Source: CAD feature listing. Evaluate the final solid. Frame: model axes, mm. A direction names the side the tool comes from. Coordinates: 2 decimals unless noted, no trailing zeros. Loops run counter-clockwise (first coordinate to the right, second up) from the corner with the lowest first, then second, coordinate; pieces in that order, holes last.
Item 1: Section query C-C, the plane y = 22. Return the cut outline in (x, z).
Item 2: Line query: probe 1 along Y at (x, z) = (0, -1.25); probe 2 along Y at (x, z) = (-20.5, 0.25); probe 3 along Y at (x, z) = (16, 1.25). Output: solid intervals per line, ascending.
Item 3: Pin query (flat end, axial travel): pin 1 Ø1.5 at (x, z) = (17.5, -1.5) entering from -Y; pin 2 Ø1 at (x, z) = (-21, -2.5) entering from +Y; pin 3 Ø3 at (y, z) = (-4, 3.5) entering from +X; pin 4 Ø1 at (y, z) = (-22, -3) entering from -X. Return the tip coordinate at first contact, or that it passes through.
Item 4: Section query B-B, the plane y = -1.5. Return the cut outline in (x, z), then the cut area to 3 significant figures.
Item 5: Reachability of faces 4 (the cylindrical face through (-4, -39.8, 0.1)), 5 (the flat face through (17.41, -21.65, 0.07)) from +Z, -Z, +X, -X, +Y, -Y: full face, straight path, thin tool, end or side. Return the list, or none.
Item 6: Pull-direction query (X, two-part tool) for faces 1 (the flat face through (-3, 27, 0)), 2 (the cylindrical face through (4, -39.8, 0.1)), 3 (the cylindrical face through (-4, 39.8, 0.1)); classes: +X half, -X half, draft (parallel to the pull), parting line (faces both ways), or undercut.
Item 7: Section query D-D, the plane x = 19.5. Return the cut outline in (y, z), then the cut area to 3 significant figures.
Item 8: Section query A-A, the plane x = 0. Return the cut outline in (y, z), then the cut area to 3 significant figures.
```python
from build123d import *

# Parameters (mm, degrees)
SKETCH1_R           = 10.5
BOSS_EXTRUDE1_DEPTH = 5


with BuildPart() as part:
    # Sketch1 → Boss-Extrude1 (new, symmetric)
    with BuildSketch(Plane.XY):
        with BuildLine():
            Line((-3, 15), (-3, 39.88734135))
            ThreePointArc((-3, 39.88734135), (-3.996245887, 39.799874608), (-4.98999373, 39.687529056))
            ThreePointArc((-4.98999373, 39.687529056), (-13.349724383, 32.229085659), (-24.534862519, 31.591779329))
            ThreePointArc((-24.534862519, 31.591779329), (-25.31698866, 30.968533792), (-26.083289209, 30.325929896))
            Line((-26.083289209, 30.325929896), (-8.485281374, 12.727922061))
            ThreePointArc((-8.485281374, 12.727922061), (-8.485281374, 8.485281374), (-12.727922061, 8.485281374))
            Line((-12.727922061, 8.485281374), (-30.325929896, 26.083289209))
            ThreePointArc((-30.325929896, 26.083289209), (-30.968533792, 25.31698866), (-31.591779329, 24.534862519))
            ThreePointArc((-31.591779329, 24.534862519), (-32.229085659, 13.349724383), (-39.687529056, 4.98999373))
            ThreePointArc((-39.687529056, 4.98999373), (-39.799874608, 3.996245887), (-39.88734135, 3))
            Line((-39.88734135, 3), (-15, 3))
            ThreePointArc((-15, 3), (-12, 0), (-15, -3))
            Line((-15, -3), (-39.88734135, -3))
            ThreePointArc((-39.88734135, -3), (-39.799874608, -3.996245887), (-39.687529056, -4.98999373))
            ThreePointArc((-39.687529056, -4.98999373), (-32.229085659, -13.349724383), (-31.591779329, -24.534862519))
            ThreePointArc((-31.591779329, -24.534862519), (-30.968533792, -25.31698866), (-30.325929896, -26.083289209))
            Line((-30.325929896, -26.083289209), (-12.727922061, -8.485281374))
            ThreePointArc((-12.727922061, -8.485281374), (-8.485281374, -8.485281374), (-8.485281374, -12.727922061))
            Line((-8.485281374, -12.727922061), (-26.083289209, -30.325929896))
            ThreePointArc((-26.083289209, -30.325929896), (-25.31698866, -30.968533792), (-24.534862519, -31.591779329))
            ThreePointArc((-24.534862519, -31.591779329), (-13.349724383, -32.229085659), (-4.98999373, -39.687529056))
            ThreePointArc((-4.98999373, -39.687529056), (-3.996245887, -39.799874608), (-3, -39.88734135))
            Line((-3, -39.88734135), (-3, -15))
            ThreePointArc((-3, -15), (0, -12), (3, -15))
            Line((3, -15), (3, -39.88734135))
            ThreePointArc((3, -39.88734135), (3.996245887, -39.799874608), (4.98999373, -39.687529056))
            ThreePointArc((4.98999373, -39.687529056), (13.349724383, -32.229085659), (24.534862519, -31.591779329))
            ThreePointArc((24.534862519, -31.591779329), (25.31698866, -30.968533792), (26.083289209, -30.325929896))
            Line((26.083289209, -30.325929896), (8.485281374, -12.727922061))
            ThreePointArc((8.485281374, -12.727922061), (8.485281374, -8.485281374), (12.727922061, -8.485281374))
            Line((12.727922061, -8.485281374), (30.325929896, -26.083289209))
            ThreePointArc((30.325929896, -26.083289209), (30.968533792, -25.31698866), (31.591779329, -24.534862519))
            ThreePointArc((31.591779329, -24.534862519), (32.229085659, -13.349724383), (39.687529056, -4.98999373))
            ThreePointArc((39.687529056, -4.98999373), (39.799874608, -3.996245887), (39.88734135, -3))
            Line((39.88734135, -3), (15, -3))
            ThreePointArc((15, -3), (12, 0), (15, 3))
            Line((15, 3), (39.88734135, 3))
            ThreePointArc((39.88734135, 3), (39.799874608, 3.996245887), (39.687529056, 4.98999373))
            ThreePointArc((39.687529056, 4.98999373), (32.229085659, 13.349724383), (31.591779329, 24.534862519))
            ThreePointArc((31.591779329, 24.534862519), (30.968533792, 25.31698866), (30.325929896, 26.083289209))
            Line((30.325929896, 26.083289209), (12.727922061, 8.485281374))
            ThreePointArc((12.727922061, 8.485281374), (8.485281374, 8.485281374), (8.485281374, 12.727922061))
            Line((8.485281374, 12.727922061), (26.083289209, 30.325929896))
            ThreePointArc((26.083289209, 30.325929896), (25.31698866, 30.968533792), (24.534862519, 31.591779329))
            ThreePointArc((24.534862519, 31.591779329), (13.349724383, 32.229085659), (4.98999373, 39.687529056))
            ThreePointArc((4.98999373, 39.687529056), (3.996245887, 39.799874608), (3, 39.88734135))
            Line((3, 39.88734135), (3, 15))
            ThreePointArc((3, 15), (0, 12), (-3, 15))
        make_face()
        Circle(SKETCH1_R, mode=Mode.SUBTRACT)
    extrude(amount=BOSS_EXTRUDE1_DEPTH, both=True)


solid = part.part
```
Verdict:
1. outline: (-31.07, -5) - (-26.24, -5) - (-26.24, 5) - (-31.07, 5) - close; (-17.76, -5) - (-3, -5) - (-3, 5) - (-17.76, 5) - close; (3, -5) - (17.76, -5) - (17.76, 5) - (3, 5) - close; (26.24, -5) - (31.07, -5) - (31.07, 5) - (26.24, 5) - close
2. probe 1: y = -12 to -10.5, 10.5 to 12
2. probe 2: y = -30.95 to -24.74, -16.26 to -3, 3 to 16.26, 24.74 to 30.95
2. probe 3: y = -31.38 to -20.24, -11.76 to -3, 3 to 11.76, 20.24 to 31.38
3. pin 1: stops at y = -31.22
3. pin 2: stops at y = 31.01
3. pin 3: stops at x = 39.89
3. pin 4: stops at x = -31.14
4. outline: (-12.4, -5) - (-10.39, -5) - (-10.39, 5) - (-12.4, 5) - close; (10.39, -5) - (12.4, -5) - (12.4, 5) - (10.39, 5) - close
4. area: 40.2 mm2
5. face 4: +Z, -Z, -X, -Y
5. face 5: +Z, -Z
6. face 1: undercut
6. face 2: +X half
6. face 3: -X half
7. outline: (-30.94, -5) - (-23.74, -5) - (-23.74, 5) - (-30.94, 5) - close; (-15.26, -5) - (-3, -5) - (-3, 5) - (-15.26, 5) - close; (3, -5) - (15.26, -5) - (15.26, 5) - (3, 5) - close; (23.74, -5) - (30.94, -5) - (30.94, 5) - (23.74, 5) - close
7. area: 389 mm2
8. outline: (-12, -5) - (-10.5, -5) - (-10.5, 5) - (-12, 5) - close; (10.5, -5) - (12, -5) - (12, 5) - (10.5, 5) - close
8. area: 30.0 mm2
